Verification items for the finished model (mm, model axes). Face numbers are marked on the shaded views. A direction names the side the tool comes from. Round coordinates to 2 decimals unless told otherwise and drop trailing zeros. Write each loop counter-clockwise with the first axis right and the second up, starting at its lowest first coordinate (ties: lowest second). Pieces come first, ordered by that corner, then holes.
from build123d import *

# Parameters (mm, degrees)
EXTRUDE_1_DEPTH = 8.89


with BuildPart() as part:
    # 草图1 → 凸台-拉伸1 (new body)
    with BuildSketch(Plane.XY):
        with BuildLine():
            Line((-15.026842649, 0), (-12.7, 0))
            ThreePointArc((-12.7, 0), (0, -12.7), (12.7, 0))
            Line((12.7, 0), (15.026842649, 0))
            ThreePointArc((15.026842649, 0), (16.966799693, -0.90043705), (17.531316424, -2.963333333))
            ThreePointArc((17.531316424, -2.963333333), (14.706844565, -9.991852829), (9.213060739, -15.206837667))
            ThreePointArc((9.213060739, -15.206837667), (8.316225051, -16.132532355), (7.989212273, -17.379243047))
            Line((7.989212273, -17.379243047), (7.989212273, -24.999243047))
            Line((7.989212273, -24.999243047), (-7.989212273, -24.999243047))
            Line((-7.989212273, -24.999243047), (-7.989212273, -17.379243047))
            ThreePointArc((-7.989212273, -17.379243047), (-8.316225051, -16.132532355), (-9.213060739, -15.206837667))
            ThreePointArc((-9.213060739, -15.206837667), (-14.706844565, -9.991852829), (-17.531316424, -2.963333333))
            ThreePointArc((-17.531316424, -2.963333333), (-16.966799693, -0.90043705), (-15.026842649, 0))
        make_face()
    extrude(amount=EXTRUDE_1_DEPTH)


solid = part.part
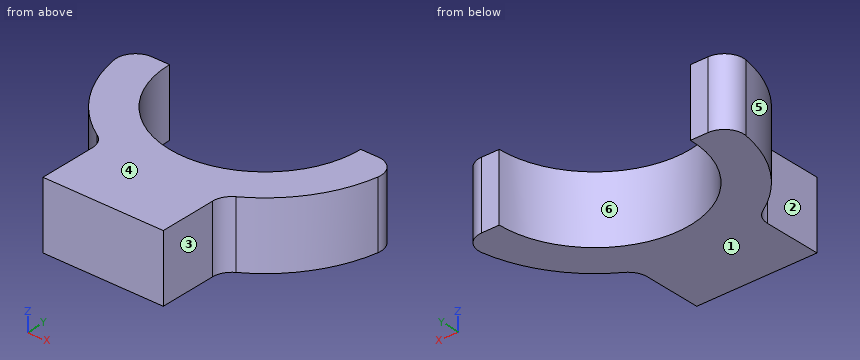
Q1. Sectioned sample at C-C (y = -18.25). Enter the section's corners in (x, z).
Recorded:
outline: (-7.99, 0) - (7.99, 0) - (7.99, 8.89) - (-7.99, 8.89) - close
Q2. Release check for a two-part mould opening along X. For the marked faces 4, 5 and 6 record: released by +X, released by -X, zero draft, split by the parting line, or undercut.
Recorded:
face 4: zero draft
face 5: released by -X
face 6: undercut
Q3. Sectioned sample at A-A (y = -4.75). Enter the section's corners in (x, z).
Recorded:
outline: (-17.13, 0) - (-11.78, 0) - (-11.78, 8.89) - (-17.13, 8.89) - close; (11.78, 0) - (17.13, 0) - (17.13, 8.89) - (11.78, 8.89) - close
Q4. Sectioned sample at D-D (x = 0). Enter the section's corners in (y, z).
Recorded:
outline: (-25, 0) - (-12.7, 0) - (-12.7, 8.89) - (-25, 8.89) - close
Q5. Depth check by flat-ended pin: P1, Ø1.5, axis at y = -20.5, z = 7.5, coming from the +X side; P2, Ø2, axis at x = 8, y = -18.5, coming from the -Z side; P3, Ø2, axis at y = -7.5, z = 6.5, coming from the -X side; P4, Ø2, axis at y = -13, z = 7.5, coming from the -X side. Enter the tip coordinate at first touch or a pass-through.
Recorded:
P1: stops at x = 7.99
P2: stops at z = 0
P3: stops at x = -16.55
P4: stops at x = -13.12
Q6. Material ranges on line 1 along X through (y, z) = (-8.5, 7.25); line 2 along X through (y, z) = (-23.5, 8.75); line 3 along X through (y, z) = (-9.5, 6.25), recorded low to high.
Recorded:
line 1: x = -15.62 to -9.44, 9.44 to 15.62
line 2: x = -7.99 to 7.99
line 3: x = -15.03 to -8.43, 8.43 to 15.03
Q7. Tool access check on the marked faces 1, 2 and 3. Record the directions out of +Z, -Z, +X, -X, +Y, -Y that give a thin tool (end or side, any length) a straight path to the whole face; none if there is none.
Recorded:
face 1: -Z, +X, -X, +Y, -Y
face 2: +Z, -Z, -X, -Y
face 3: +Z, -Z, +X, -Y
Q8. Sectioned sample at B-B (z = 2). Enter the section's corners in (x, y).
Recorded:
outline: (-17.53, -2.96) arc R17.78 ccw to (-9.21, -15.21) arc R2.54 cw to (-7.99, -17.38) - (-7.99, -25) - (7.99, -25) - (7.99, -17.38) arc R2.54 cw to (9.21, -15.21) arc R17.78 ccw to (17.53, -2.96) arc R2.54 ccw to (15.03, 0) - (12.7, 0) arc R12.7 cw to (-12.7, 0) - (-15.03, 0) arc R2.54 ccw to start
